Answer from the drawing. Dimensions are ordinates in mm from the lowest x, y and z of the part. A direction names the side the tool comes from. Coordinates: 2 decimals unless noted, no trailing zeros. Loops run counter-clockwise (first coordinate to the right, second up) from the corner with the lowest first, then second, coordinate; pieces in that order, holes last. Notation, with made-up numbers: (2, 19.5) -> (20, 19.5) arc R31 ccw to (20, 56.5) -> close; hole circle Ø2 at (-23, -17). An arc over 180 degrees is marked (long way). Answer as CSV lines item,"result".
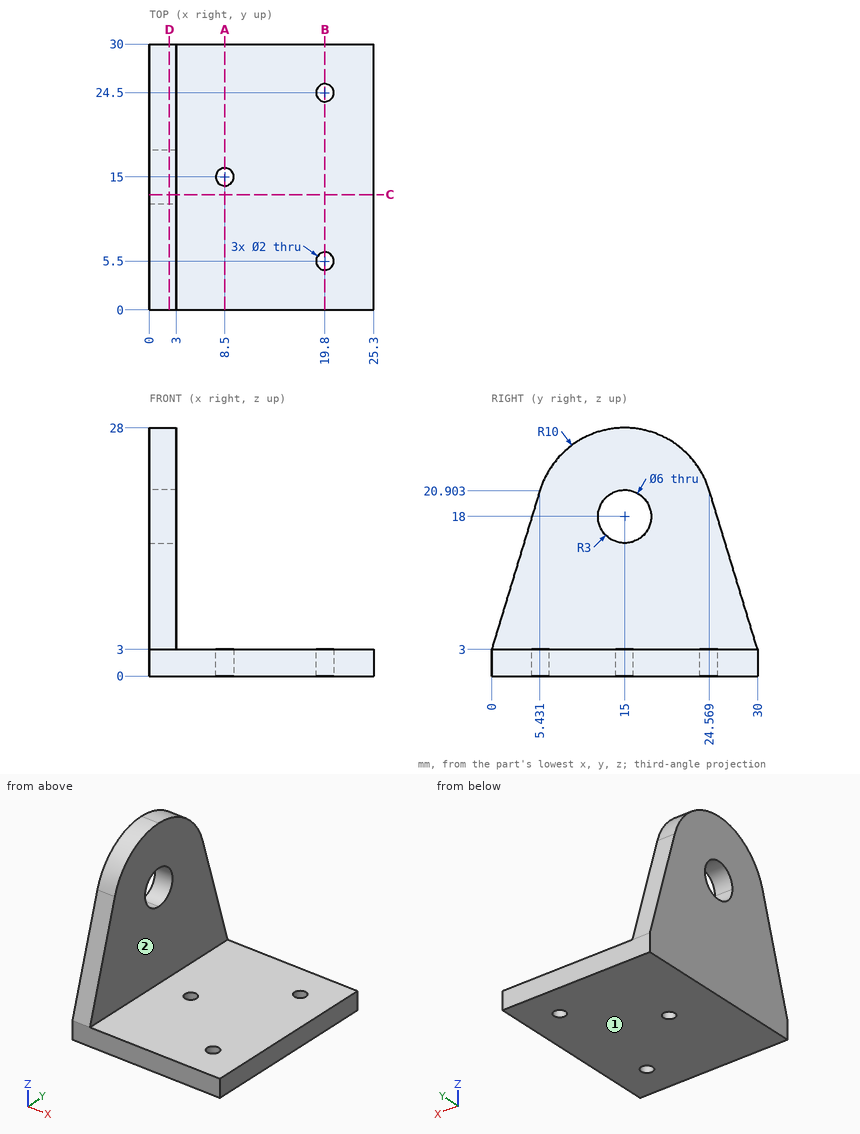
(1) A cutting plane is placed at D-D, the plane x = 2.25. Write down the section's boundary in (y, z).
Computed values:
outline,"(0, 0) -> (30, 0) -> (30, 3) -> (24.57, 20.9) arc R10 ccw to (5.43, 20.9) -> (0, 3) -> close; hole circle Ø6 at (15, 18)"
(2) A cutting plane is placed at C-C, the plane y = 13. Write down the section's boundary in (x, z).
Computed values:
outline,"(0, 0) -> (25.3, 0) -> (25.3, 3) -> (3, 3) -> (3, 15.76) -> (0, 15.76) -> close; (0, 20.24) -> (3, 20.24) -> (3, 27.8) -> (0, 27.8) -> close"
(3) Flat-ended cylindrical pins translate along their axes: pin 1 Ø1 at (x, y) = (22.5, 8) entering from +Z; pin 2 Ø1.8 at (x, y) = (19.8, 5.5) entering from +Z; pin 3 Ø3 at (y, z) = (5, 15) entering from +X. Find the tip coordinate at first contact, or state that the pin passes through.
Computed values:
pin 1,"z = 3"
pin 2,"through"
pin 3,"x = 3"
(4) Which of the six approach directions +Z, -Z, +X, -X, +Y, -Y give full straight-line access (tool end or side, diameter ignored) to the marked faces 1 and 2?
Computed values:
face 1,"-Z, +X, -X, +Y, -Y"
face 2,"+Z, +X, +Y, -Y"
(5) A cutting plane is placed at A-A, the plane x = 8.5. Write down the section's boundary in (y, z).
Computed values:
outline,"(0, 0) -> (14, 0) -> (14, 3) -> (0, 3) -> close; (16, 0) -> (30, 0) -> (30, 3) -> (16, 3) -> close"
(6) A cutting plane is placed at B-B, the plane x = 19.8. Write down the section's boundary in (y, z).
Computed values:
outline,"(0, 0) -> (4.5, 0) -> (4.5, 3) -> (0, 3) -> close; (6.5, 0) -> (23.5, 0) -> (23.5, 3) -> (6.5, 3) -> close; (25.5, 0) -> (30, 0) -> (30, 3) -> (25.5, 3) -> close"
(7) Consider line 1 along Y through (x, z) = (19.8, 2); line 2 along Z through (x, y) = (12.5, 18.5); line 3 along Y through (x, z) = (1.5, 18). Determine where each line is inside the solid, lowest interval first.
Computed values:
line 1,"0 to 4.5, 6.5 to 23.5, 25.5 to 30"
line 2,"0 to 3"
line 3,"4.55 to 12, 18 to 25.45"
